from build123d import *

# Parameters (mm, degrees)
SKETCH2_R           = 2.5
BOSS_EXTRUDE1_DEPTH = 3
SKETCH3_W           = 30
SKETCH3_H           = 30
BOSS_EXTRUDE2_DEPTH = 40
CUT_EXTRUDE2_DEPTH  = 30
CUT_EXTRUDE3_DEPTH  = 30
SKETCH12_W          = 3.1
SKETCH12_H          = 30
SKETCH12_W_2        = 8.45
SKETCH12_W_3        = 10.45
CUT_EXTRUDE4_DEPTH  = 20
SKETCH13_R          = 2.5
CUT_EXTRUDE5_DEPTH  = 15
CUT_EXTRUDE6_DEPTH  = 3


with BuildPart() as part:
    # Sketch2 → Boss-Extrude1 (new body)
    with BuildSketch(Plane(origin=(0, 0, 0), x_dir=(1, 0, 0), z_dir=(0, 1, 0))):
        with BuildLine():
            Line((-26, -30), (26, -30))
            ThreePointArc((26, -30), (28.828427125, -28.828427125), (30, -26))
            Line((30, -26), (30, 26))
            ThreePointArc((30, 26), (28.828427125, 28.828427125), (26, 30))
            Line((26, 30), (-26, 30))
            ThreePointArc((-26, 30), (-28.828427125, 28.828427125), (-30, 26))
            Line((-30, 26), (-30, -26))
            ThreePointArc((-30, -26), (-28.828427125, -28.828427125), (-26, -30))
        make_face()
        with Locations(Location((-24.1, 25, 0), (0, 0, 270))):
            Circle(SKETCH2_R, mode=Mode.SUBTRACT)
        with Locations(Location((24.1, 25, 0), (0, 0, 270))):
            Circle(SKETCH2_R, mode=Mode.SUBTRACT)
        with Locations(Location((-24.1, -25, 0), (0, 0, 270))):
            Circle(SKETCH2_R, mode=Mode.SUBTRACT)
        with Locations(Location((24.1, -25, 0), (0, 0, 270))):
            Circle(SKETCH2_R, mode=Mode.SUBTRACT)
    extrude(amount=BOSS_EXTRUDE1_DEPTH)

    # Sketch3 → Boss-Extrude2 (add)
    with BuildSketch(Plane(origin=(0, 3, 0), x_dir=(1, 0, 0), z_dir=(0, 1, 0))):
        Rectangle(SKETCH3_W, SKETCH3_H)
    extrude(amount=BOSS_EXTRUDE2_DEPTH)

    # Sketch8 → Cut-Extrude2 (cut)
    with BuildSketch(Plane(origin=(15, 0, 0), x_dir=(0, 0, -1), z_dir=(1, 0, 0))):
        with BuildLine():
            Line((-7.317073171, 37.146341463), (-15, 3))
            Line((-15, 3), (-15, 43))
            Line((-15, 43), (0, 43))
            ThreePointArc((0, 43), (-4.685212857, 41.356516071), (-7.317073171, 37.146341463))
        make_face()
    extrude(amount=-CUT_EXTRUDE2_DEPTH, mode=Mode.SUBTRACT)

    # Sketch10 → Cut-Extrude3 (cut)
    with BuildSketch(Plane(origin=(15, 0, 0), x_dir=(0, 0, -1), z_dir=(1, 0, 0))):
        with BuildLine():
            Line((7.317073171, 37.146341463), (15, 3))
            Line((15, 3), (15, 43))
            Line((15, 43), (0, 43))
            ThreePointArc((0, 43), (4.685212857, 41.356516071), (7.317073171, 37.146341463))
        make_face()
    extrude(amount=-CUT_EXTRUDE3_DEPTH, mode=Mode.SUBTRACT)

    # Sketch12 → Cut-Extrude4 (cut, symmetric)
    with BuildSketch(Plane(origin=(0, 23, 0), x_dir=(1, 0, 0), z_dir=(0, 1, 0))):
        Rectangle(SKETCH12_W, SKETCH12_H)
        with Locations((-10.775, 0)):
            Rectangle(SKETCH12_W_2, SKETCH12_H)
        with Locations((9.775, 0)):
            Rectangle(SKETCH12_W_3, SKETCH12_H)
    extrude(amount=CUT_EXTRUDE4_DEPTH, both=True, mode=Mode.SUBTRACT)

    # Sketch13 → Cut-Extrude5 (cut, symmetric)
    with BuildSketch(Plane(origin=(0, 0, 0), x_dir=(0, 0, -1), z_dir=(1, 0, 0))):
        with Locations((0, 35.5)):
            Circle(SKETCH13_R)
    extrude(amount=CUT_EXTRUDE5_DEPTH, both=True, mode=Mode.SUBTRACT)

    # Sketch14 → Cut-Extrude6 (cut)
    with BuildSketch(Plane.ZY.offset(6.55)):
        Polygon((-3.507402885, 37.525), (-3.507402885, 33.475), (0, 31.45), (3.507402885, 33.475), (3.507402885, 37.525), (0, 39.55), align=None)
    extrude(amount=-CUT_EXTRUDE6_DEPTH, mode=Mode.SUBTRACT)


solid = part.part
Input: part model. Units: mm. Frame: model coordinates. A direction names the side the tool comes from. Round coordinates to 2 decimals unless told otherwise and drop trailing zeros. Write each loop counter-clockwise with the first axis right and the second up, starting at its lowest first coordinate (ties: lowest second). Pieces come first, ordered by that corner, then holes.
1) Cut plane A-A (z = 25). Return the cut outline in (x, y), then the cut area to 3 significant figures.
2) Cut plane B-B (y = 15). Return the cut outline in (x, z).
3) Cut plane D-D (z = 6). Return the cut outline in (x, y).
4) Contact query for flat-ended pins moving along their axis: P1, Ø24, axis at y = 21.5, z = 3.5, coming from the -X side; P2, Ø4, axis at y = 35.5, z = 0, coming from the +X side; P3, Ø0.9, axis at x = -4.5, y = 35, coming from the +Z side; P4, Ø3.5, axis at y = 35, z = -1.5, coming from the -X side. Output: stop coordinate, or through.
5) Draft query along Z for faces 5 (the flat face through (0, 1, 30)), 6 (the flat face through (0, 1, -30)), 7 (the flat face through (-30, 1, 0)), 8 (the cylindrical face through (-22.41, 1.48, -26.84)). Return one class per face: pulls with the +Z half, pulls with the -Z half, needs draft (parallel to the pull), parting line crosses it, or undercut.
6) Ray query, L1, parallel to X at y = 1.15, z = -25; L2, parallel to Z at x = 24, y = 1; L3, parallel to Y at x = 3.25, z = 0. Return the intervals inside material, ascending.
7) Cut plane C-C (x = 24.1). Return the cut outline in (y, z).
8) Reachability of faces 1 (the flat face through (-6.55, 18, 0)), 2 (the flat face through (1.55, 18, 0)), 3 (the flat face through (-5.07, 38.55, -1.73)), 4 (the flat face through (4.55, 19, 0)) from +Z, -Z, +X, -X, +Y, -Y: full face, straight path, thin tool, end or side. Return the list, or none.
Geometry says:
1. outline: (-30, 0) - (-26.6, 0) - (-26.6, 3) - (-30, 3) - close; (-21.6, 0) - (21.6, 0) - (21.6, 3) - (-21.6, 3) - close; (26.6, 0) - (30, 0) - (30, 3) - (26.6, 3) - close
1. area: 150 mm2
2. outline: (-6.55, -12.3) - (-1.55, -12.3) - (-1.55, 12.3) - (-6.55, 12.3) - close; (1.55, -12.3) - (4.55, -12.3) - (4.55, 12.3) - (1.55, 12.3) - close
3. outline: (-30, 0) - (30, 0) - (30, 3) - (4.55, 3) - (4.55, 40) - (1.55, 40) - (1.55, 3) - (-1.55, 3) - (-1.55, 40) - (-6.55, 40) - (-6.55, 3) - (-30, 3) - close
4. P1: stops at x = -6.55
4. P2: passes through
4. P3: stops at z = 7.9
4. P4: stops at x = -3.55
5. face 5: pulls with the +Z half
5. face 6: pulls with the -Z half
5. face 7: needs draft
5. face 8: undercut
6. L1: x = -30 to -26.6, -21.6 to 21.6, 26.6 to 30
6. L2: z = -30 to -27.5, -22.5 to 22.5, 27.5 to 30
6. L3: y = 0 to 33, 38 to 43
7. outline: (0, -30) - (3, -30) - (3, -27.5) - (0, -27.5) - close; (0, -22.5) - (3, -22.5) - (3, 22.5) - (0, 22.5) - close; (0, 27.5) - (3, 27.5) - (3, 30) - (0, 30) - close
8. face 1: +Z, -Z, -X, +Y
8. face 2: +Z, -Z, +Y
8. face 3: -X
8. face 4: +Z, -Z, +X, +Y
